```python
from build123d import *

# Parameters (mm, degrees)
F0_W      = 70
F0_H      = 15
F1_DEPTH  = 8.75
F2_W      = 70
F2_H      = 30
F3_DEPTH  = 5
F4_W      = 70
F4_H      = 15
F5_DEPTH  = 15
F6_W      = 5
F6_H      = 5
F8_R      = 10
F9_DEPTH  = 3
F10_R     = 10
F11_DEPTH = 3
F12_R     = 10
F13_DEPTH = 3
F14_R     = 2.5
F15_DEPTH = 3
F16_R     = 2.5
F17_DEPTH = 3
F18_R     = 2.5
F19_DEPTH = 3
F20_R     = 2.5
F21_DEPTH = 3
F23_DEPTH = 15
F24_R     = 5
F25_R     = 5


# Not quite as in the source:
# - a pattern or mirror of a feature is missing from the dataset's text; its kind, count and spacing are read off the source's solid


with BuildPart() as f1:
    # F0 (on Top) → F1 (new body, symmetric)
    with BuildSketch(Plane.XY):
        Rectangle(F0_W, F0_H)
    extrude(amount=F1_DEPTH, both=True)

    # F2 (on face) → F3 (join)
    with BuildSketch(Plane.XY.offset(8.75)):
        Rectangle(F2_W, F2_H)
    extrude(amount=F3_DEPTH)

    # F4 (on face) → F5 (join)
    with BuildSketch(Plane.XY.offset(13.75)):
        Rectangle(F4_W, F4_H)
    extrude(amount=F5_DEPTH)

    # F6 (on Front) → F7 (revolve)
    with BuildSketch(Plane.XZ):
        with Locations((-37.5, -2.5)):
            Rectangle(F6_W, F6_H)
    revolve(axis=Axis((0.3605282434, 0, 0), (1, 0, 0)))

    # F8 (on face) → F9 (join)
    with BuildSketch(Plane.XZ.offset(7.5)):
        with Locations((-22.5, -3.75)):
            Circle(F8_R)
    f9 = extrude(amount=F9_DEPTH)

    # F9_copies: F9 across plane
    add(f9.mirror(Plane.ZX))

    # F10 (on face) → F11 (join)
    with BuildSketch(Plane.XZ.offset(7.5)):
        with Locations((0, -3.75)):
            Circle(F10_R)
    f11 = extrude(amount=F11_DEPTH)

    # F11_copies: F11 across plane
    add(f11.mirror(Plane.ZX))

    # F12 (on face) → F13 (join)
    with BuildSketch(Plane.XZ.offset(7.5)):
        with Locations((22.5, -3.75)):
            Circle(F12_R)
    f13 = extrude(amount=F13_DEPTH)

    # F13_copies: F13 across plane
    add(f13.mirror(Plane.ZX))

    # F14 (on face) → F15 (join)
    with BuildSketch(Plane.XZ.offset(10.5)):
        with Locations((-22.5, -3.75)):
            Circle(F14_R)
    f15 = extrude(amount=F15_DEPTH)

    # F15_copies: F15 across plane
    add(f15.mirror(Plane.ZX))

    # F16 (on face) → F17 (join)
    with BuildSketch(Plane.XZ.offset(10.5)):
        with Locations((0, -3.75)):
            Circle(F16_R)
    f17 = extrude(amount=F17_DEPTH)

    # F17_copies: F17 across plane
    add(f17.mirror(Plane.ZX))

    # F18 (on face) → F19 (join)
    with BuildSketch(Plane.XZ.offset(10.5)):
        with Locations((22.5, -3.75)):
            Circle(F18_R)
    f19 = extrude(amount=F19_DEPTH)

    # F19_copies: F19 across plane
    add(f19.mirror(Plane.ZX))

    # F20 (on face) → F21 (join)
    with BuildSketch(Plane.XY.offset(28.75)):
        with Locations((20, 0)):
            Circle(F20_R)
    extrude(amount=F21_DEPTH)

    # F22 (on face) → F23 (cut, through all)
    with BuildSketch(Plane.XZ.offset(7.5)):
        Polygon((-12.5, 28.75), (-27.5, 28.75), (-24.5953480316, 24.6802337976), (-17.5, 22.25), (-17.5, 21.25), (-12.5, 21.25), align=None)
    extrude(amount=-F23_DEPTH, mode=Mode.SUBTRACT)

    # F24
    f24_edges = [f1.edges().sort_by_distance(p)[0] for p in [
        (11.25, -7.5, 28.75),
        (11.25, 7.5, 28.75),
    ]]
    fillet(f24_edges, radius=F24_R)

    # F25
    f25_edges = [f1.edges().sort_by_distance(p)[0] for p in [
        (-31.25, -7.5, 28.75),
        (-31.25, 7.5, 28.75),
    ]]
    fillet(f25_edges, radius=F25_R)

    # F26 (on Front) → F27 (revolve)
    with BuildSketch(Plane.XZ):
        with BuildLine():
            Line((-40, 0), (-40, 5))
            ThreePointArc((-40, 5), (-43.5355339059, 3.5355339059), (-45, 0))
            Line((-45, 0), (-40, 0))
        make_face()
    revolve(axis=Axis((-36.5614034235, 0, 0), (1, 0, 0)))


solid = f1.part
```
Input: part model. Units: mm. Frame: model coordinates. A direction names the side the tool comes from. Coordinates: 2 decimals unless noted, no trailing zeros. Write each loop counter-clockwise with the first axis right and the second up, starting at its lowest first coordinate (ties: lowest second). Pieces come first, ordered by that corner, then holes.
1) Pin query (flat end, axial travel): pin 1 Ø16 at (x, z) = (3.5, -4.5) entering from +Y; pin 2 Ø1.5 at (x, z) = (26, -12) entering from -Y; pin 3 Ø4 at (x, z) = (-19, -11) entering from +Y. Return the tip coordinate at first contact, or that it passes through.
2) Material intervals for line 1 along X through (y, z) = (7.75, -4); line 2 along Y through (x, z) = (25, -9); line 3 along Z through (x, y) = (22.5, -9.5), sorted ascending.
3) Mould query, pull axis Y, two halves, no side actions, for faces 1 (the flat face through (0, 7.5, -11)), 2 (the flat face through (-26.068, -0.104, 26.744)), 3 (the flat face through (-23, -7.5, -11)), 4 (the flat face through (22, 13.5, -4)). Classes: pulls with the +Y half, pulls with the -Y half, needs draft (parallel to the pull), parting line crosses it, or undercut.
4) Section B-B on y = 0. Output: boundary loops of the cut face in (x, z), and give its area (3 significant figures).
5) Set-up query: faces 5 (the flat face through (0, -11, 8.75)), 6 (the cylindrical face through (-37.47, -4.88, 1.08)), 7 (the cylindrical face through (-12.96, -8.98, -0.75)). Return all of +Z, -Z, +X, -X, +Y, -Y with unobstructed straight access to the full face (end or side cutting, diameter ignored); none if empty.
6) Section A-A on z = 26.5. Output: boundary loops of the cut face in (x, y), and give its area (3 significant figures).
Check result:
1. pin 1: stops at y = 13.5
1. pin 2: stops at y = -10.5
1. pin 3: stops at y = 10.5
2. line 1: x = -32.5 to -12.5, -10 to 10, 12.5 to 32.5
2. line 2: y = -10.5 to -7.5, 7.5 to 10.5
2. line 3: z = -13.75 to 6.25, 8.75 to 13.75
3. face 1: undercut
3. face 2: needs draft
3. face 3: undercut
3. face 4: pulls with the +Y half
4. outline: (-40, -5) - (-35, -5) - (-35, -8.75) - (35, -8.75) - (35, 28.75) - (22.5, 28.75) - (22.5, 31.75) - (17.5, 31.75) - (17.5, 28.75) - (-12.5, 28.75) - (-12.5, 21.25) - (-17.5, 21.25) - (-17.5, 22.25) - (-24.6, 24.68) - (-27.5, 28.75) - (-35, 28.75) - (-35, 5) - (-40, 5) arc R5 ccw to start
4. area: 2,650 mm2
5. face 5: +X, -X, -Y
5. face 6: -X
5. face 7: -Y
6. outline: (-35, -6.68) - (-25.89, -6.68) - (-25.89, 6.68) - (-35, 6.68) - close; (-12.5, -6.68) - (35, -6.68) - (35, 6.68) - (-12.5, 6.68) - close
6. area: 756 mm2
